For this review, take the finished solid that the model builds, in its own axes (mm). Coordinates: 2 decimals unless noted, no trailing zeros. Loops run counter-clockwise (first coordinate to the right, second up) from the corner with the lowest first, then second, coordinate; pieces in that order, holes last. Notation, with made-up numbers: (-31.75, 50.5) -> (-8.75, 50.5) arc R24 ccw to (-8.75, 82.5) -> close; hole circle Ø7 at (-27, -4.75). An arc over 180 degrees is marked (long way). Answer in a Markdown table with one row per item.
from build123d import *

# Parameters (mm, degrees)
F1_DEPTH = 15.875
F3_D     = 6.35
F3_DEPTH = 7.9375
F3_TIP   = 1.9077324654
F5_D     = 7.9502


with BuildPart() as f1:
    # F0 (on Front) → F1 (new body)
    with BuildSketch(Plane.XZ):
        Polygon((0, 85.598), (0, 0), (15.875, 0), (15.875, 120.65), (6.1722, 120.65), align=None)
    extrude(amount=F1_DEPTH)

    # F3
    with Locations(Plane.YZ.offset(15.875)):
        with Locations((-7.9375, 12.7508)):
            Hole(F3_D / 2, depth=F3_DEPTH)
            with Locations((0, 0, -(F3_DEPTH + F3_TIP / 2))):  # 118° drill point
                Cone(0, F3_D / 2, F3_TIP, mode=Mode.SUBTRACT)

    # F5 (through all)
    with Locations(Plane.YZ.offset(15.875)):
        with Locations((-7.9375, 70.6882)):
            Hole(F5_D / 2)


solid = f1.part
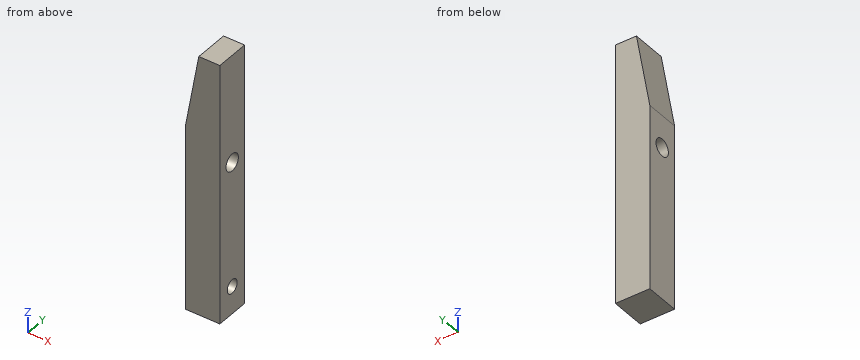
Item 1: Take a section at A-A, the plane y = -2.5. State the section outline as (x, z) points (3 decimals).
Worked answers:
| item | result |
|---|---|
| outline | (0, 0) -> (15.875, 0) -> (15.875, 120.65) -> (6.172, 120.65) -> (0, 85.598) -> close |
Item 2: Take a section at C-C, the plane z = 113.5. State the section outline as (x, y) points (3 decimals).
Worked answers:
| item | result |
|---|---|
| outline | (4.913, -15.875) -> (15.875, -15.875) -> (15.875, 0) -> (4.913, 0) -> close |
Item 3: For L1, parallel to Z at x = 10, y = -5.75; L2, parallel to Z at x = 8.25, y = -10.5; L3, parallel to Z at x = 6.5, y = -6, list the stretches that pass through material, from the lowest coordinate up.
Worked answers:
| item | result |
|---|---|
| L1 | 0 to 10.45, 15.05 to 67.37, 74.01 to 120.65 |
| L2 | 0 to 10.88, 14.63 to 67.65, 73.73 to 120.65 |
| L3 | 0 to 67.22, 74.16 to 120.65 |
Item 4: Take a section at D-D, the plane x = 14.75. Count the separate pieces of the cut face and the enclosed holes in it, and give its area (3 significant figures).
Worked answers:
| item | result |
|---|---|
| separate pieces | 1 |
| enclosed holes | 2 |
| area | 1,830 mm² |
Item 5: Insertion check: pin 1 (4 mm diameter, centred on y = -7.94, z = 12.75, fed in from +X); pin 2 (5 mm diameter, centred on y = -7.5, z = 88.5, fed in from -X). Each pin has a flat end and moves straight along its axis. Give the tip position at first contact, or say it passes through.
Worked answers:
| item | result |
|---|---|
| pin 1 | x = 7.23 |
| pin 2 | x = 0.07 |
Item 6: Take a section at B-B, the plane x = 2.25. State the section outline as (y, z) points (1 decimal).
Worked answers:
| item | result |
|---|---|
| outline | (-15.9, 0) -> (0, 0) -> (0, 98.4) -> (-15.9, 98.4) -> close; hole circle Ø8 at (-7.9, 70.7) |
